Verification items for this drawing (mm, ordinates from the low corner). A direction names the side the tool comes from. Coordinates: 2 decimals unless noted, no trailing zeros. Order: outer loops, then holes, each group sorted by start corner. A loop starts at its lowest first (then second) coordinate and runs counter-clockwise, first axis right, second up. Notation, with made-up numbers: (32, 60.25) -> (57, 60.25) arc R23 cw to (57, 82.25) -> close; hole circle Ø9 at (65, -14). An arc over 180 degrees is marked (long way). Put each result on its own line as item: value. Start each with the question number.
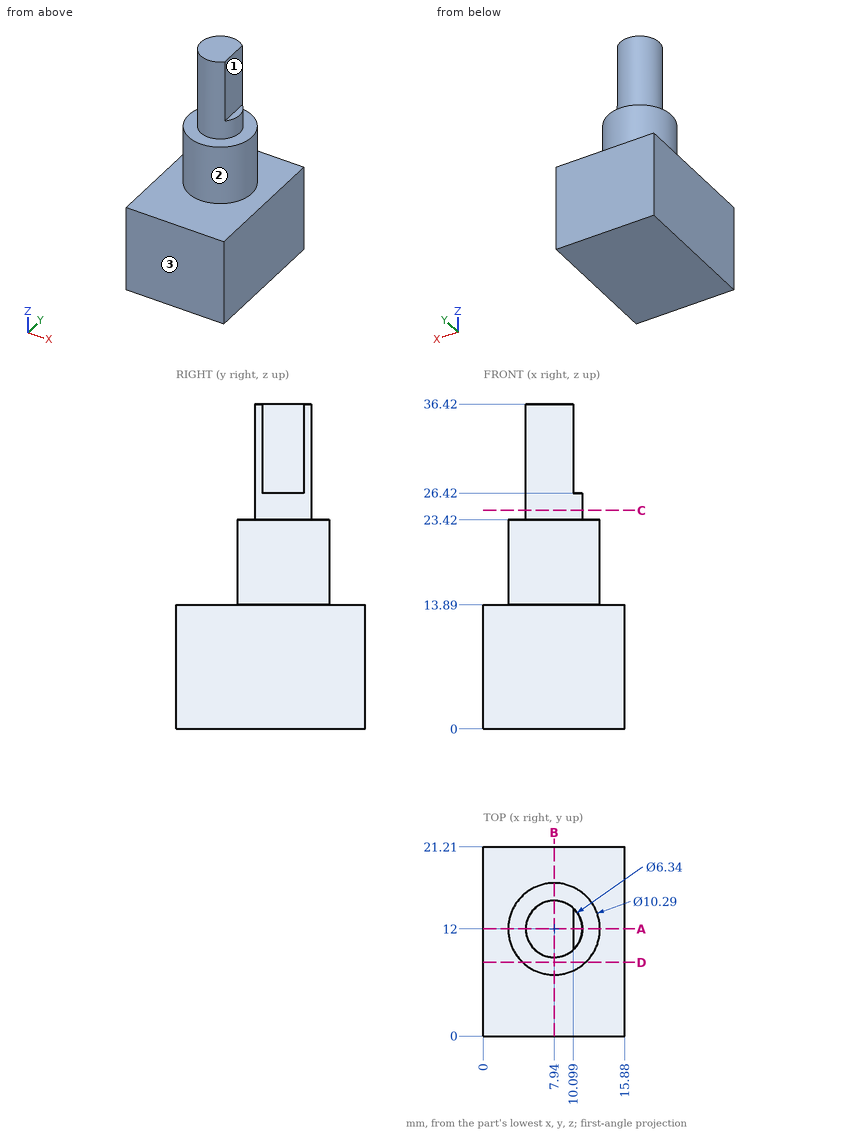
1) Gauge pin test, flat ends, axial feed: pin 1 (6 mm diameter, centred on x = 4.5, z = 26, fed in from -Y); pin 2 (2 mm diameter, centred on x = 12.5, z = 19, fed in from -Y); pin 3 (1 mm diameter, centred on y = 16.5, z = 16, fed in from -X). Record the tip position at first contact, or that the pin passes through.
2) Sectioned sample at D-D (y = 8.25). Record the boundary of the cut face in (x, z), plus the area to 3 significant figures.
3) Sectioned sample at C-C (z = 24.5). Record the boundary of the cut face in (x, y).
4) Access from +Z, -Z, +X, -X, +Y, -Y to the whole of each face (thin tool, end or side, straight path). Record for the marked faces 1, 2 and 3.
5) Sectioned sample at B-B (x = 7.94). Record the boundary of the cut face in (y, z) (3 decimals), plus the area to 3 significant figures.
6) Scan lines: line 1 along Z through (x, y) = (13.25, 12); line 2 along Y through (x, z) = (8, 22); line 3 along Z through (x, y) = (11.75, 10.25). Record each from-to range of solid material in increasing order. Write a range as [from, to].
7) Sectioned sample at A-A (y = 12). Record the boundary of the cut face in (x, z) (3 decimals).
Entries:
1. pin 1: stops at y = 7.22
1. pin 2: stops at y = 8.29
1. pin 3: stops at x = 4.7
2. outline: (0, 0) -> (15.88, 0) -> (15.88, 13.89) -> (11.46, 13.89) -> (11.46, 23.42) -> (4.42, 23.42) -> (4.42, 13.89) -> (0, 13.89) -> close
2. area: 288 mm2
3. outline: circle Ø6.34 at (7.94, 12)
4. face 1: +Z, +X, +Y, -Y
4. face 2: +Z
4. face 3: +Z, -Z, +X, -X, -Y
5. outline: (0, 0) -> (21.21, 0) -> (21.21, 13.89) -> (17.145, 13.89) -> (17.145, 23.42) -> (15.17, 23.42) -> (15.17, 36.42) -> (8.83, 36.42) -> (8.83, 23.42) -> (6.855, 23.42) -> (6.855, 13.89) -> (0, 13.89) -> close
5. area: 475 mm2
6. line 1: z = [0, 13.89]
6. line 2: y = [6.86, 17.14]
6. line 3: z = [0, 23.42]
7. outline: (0, 0) -> (15.88, 0) -> (15.88, 13.89) -> (13.085, 13.89) -> (13.085, 23.42) -> (11.11, 23.42) -> (11.11, 26.42) -> (10.099, 26.42) -> (10.099, 36.42) -> (4.77, 36.42) -> (4.77, 23.42) -> (2.795, 23.42) -> (2.795, 13.89) -> (0, 13.89) -> close
